Could you check a few things on this drawing? It's one solid part, dimensions in mm from its lowest x, y, z. Give positions to 0.01 mm unless a question says otherwise; leave off trailing zeros. Loops run counter-clockwise (first coordinate to the right, second up) from the corner with the lowest first, then second, coordinate; pieces in that order, holes last. Notation, with made-up numbers: (28, 30) - (39, 30) arc R6 cw to (39, 38) - close; hole circle Ø3 at (-12, -20). An arc over 180 degrees is marked (long way). Return JSON: item names as keys, results as strings. Group by question number.
(1) If we section it at C-C (x = 111): Please give me the cut outline in (y, z) (1 decimal).
(2) If we section it at A-A (z = 2.4): Please give me the cut outline in (x, y) (1 decimal), then the cut area to 3 significant figures.
(3) For P1, Ø1, axis at y = 27, z = 1, coming from the -X side; P2, Ø1, axis at x = 5.5, z = 1, coming from the +Y side, each with a flat end and sliding along its axis, tell me the tip position at first contact or that it passes through.
(4) If we section it at B-B (y = 12.7): Please give me the cut outline in (x, z) (1 decimal), then the cut area to 3 significant figures.
(5) I need wall thicknesses on probe 1 along X at (y, z) = (26, 0.25); probe 2 along X at (y, z) = (14.5, 2.65) (1 decimal); probe 3 along X at (y, z) = (10.75, 0.5) (1 decimal). Which ranges of each line are inside material? Lowest first, please. Write a range as [from, to].
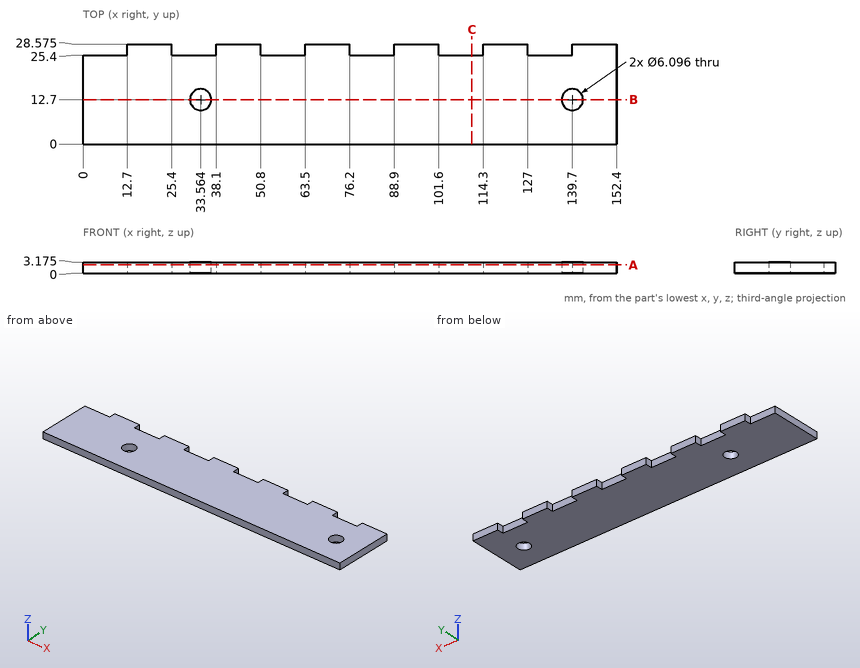
Values:
{
 "1": {"outline": "(0, 0) - (25.4, 0) - (25.4, 3.2) - (0, 3.2) - close"},
 "2": {"outline": "(0, 0) - (152.4, 0) - (152.4, 28.6) - (139.7, 28.6) - (139.7, 25.4) - (127, 25.4) - (127, 28.6) - (114.3, 28.6) - (114.3, 25.4) - (101.6, 25.4) - (101.6, 28.6) - (88.9, 28.6) - (88.9, 25.4) - (76.2, 25.4) - (76.2, 28.6) - (63.5, 28.6) - (63.5, 25.4) - (50.8, 25.4) - (50.8, 28.6) - (38.1, 28.6) - (38.1, 25.4) - (25.4, 25.4) - (25.4, 28.6) - (12.7, 28.6) - (12.7, 25.4) - (0, 25.4) - close; hole circle Ø6.1 at (33.6, 12.7); hole circle Ø6.1 at (139.7, 12.7)", "area": "4,050 mm2"},
 "3": {"P1": "x = 12.7", "P2": "y = 25.4"},
 "4": {"outline": "(0, 0) - (30.5, 0) - (30.5, 3.2) - (0, 3.2) - close; (36.6, 0) - (136.7, 0) - (136.7, 3.2) - (36.6, 3.2) - close; (142.7, 0) - (152.4, 0) - (152.4, 3.2) - (142.7, 3.2) - close", "area": "445 mm2"},
 "5": {"probe 1": "[12.7, 25.4], [38.1, 50.8], [63.5, 76.2], [88.9, 101.6], [114.3, 127], [139.7, 152.4]", "probe 2": "[0, 31.1], [36, 137.2], [142.2, 152.4]", "probe 3": "[0, 31.2], [35.9, 137.4], [142, 152.4]"}
}
